```python
from build123d import *

# Parameters (mm, degrees)
SKETCH1_R           = 2.1
BOSS_EXTRUDE1_DEPTH = 3
CUT_EXTRUDE1_DEPTH  = 3
SKETCH3_R           = 5
SKETCH3_R_2         = 2.1
BOSS_EXTRUDE2_DEPTH = 6


with BuildPart() as part:
    # Sketch1 → Boss-Extrude1 (new, symmetric)
    with BuildSketch(Plane(origin=(0, 0, 0), x_dir=(1, 0, 0), z_dir=(0, 1, 0))):
        with BuildLine():
            Line((-5, 5), (5, 5))
            ThreePointArc((5, 5), (10, 0), (5, -5))
            Line((5, -5), (-5, -5))
            ThreePointArc((-5, -5), (-10, 0), (-5, 5))
        make_face()
        with Locations(Location((5, 0, 0), (0, 0, 270))):
            Circle(SKETCH1_R, mode=Mode.SUBTRACT)
        with Locations(Location((-5, 0, 0), (0, 0, 270))):
            Circle(SKETCH1_R, mode=Mode.SUBTRACT)
    extrude(amount=BOSS_EXTRUDE1_DEPTH, both=True)

    # Sketch2 → Cut-Extrude1 (cut)
    with BuildSketch(Plane(origin=(0, 3, 0), x_dir=(1, 0, 0), z_dir=(0, 1, 0))):
        Polygon((-9.041451884, 0), (-7.020725942, -3.5), (-2.979274058, -3.5), (-0.958548116, 0), (-2.979274058, 3.5), (-7.020725942, 3.5), align=None)
        Polygon((9.041451884, 0), (7.020725942, 3.5), (2.979274058, 3.5), (0.958548116, 0), (2.979274058, -3.5), (7.020725942, -3.5), align=None)
    extrude(amount=-CUT_EXTRUDE1_DEPTH, mode=Mode.SUBTRACT)

    # Sketch3 → Boss-Extrude2 (add)
    with BuildSketch(Plane.XZ.offset(3)):
        with Locations(Location((5, 0, 0), (0, 0, 270))):
            Circle(SKETCH3_R)
        with Locations(Location((5, 0, 0), (0, 0, 270))):
            Circle(SKETCH3_R_2, mode=Mode.SUBTRACT)
    extrude(amount=BOSS_EXTRUDE2_DEPTH)


solid = part.part
```
Here's how the part is built. I have some questions about the finished solid (model axes, mm). A direction names the side the tool comes from. Give positions to 0.01 mm unless a question says otherwise; leave off trailing zeros. Write each loop counter-clockwise with the first axis right and the second up, starting at its lowest first coordinate (ties: lowest second). Pieces come first, ordered by that corner, then holes. Notation, with made-up numbers: (-11.5, 80.25) -> (14.5, 80.25) arc R29 ccw to (14.5, 102.25) -> close; hole circle Ø11 at (84, 32.5). An arc over 180 degrees is marked (long way). Write each question's results on one line, items separated by ' | '.
Item 1: If I drill on L1, parallel to X at y = -0.85, z = 0; L2, parallel to Z at x = -5, y = -1.9; L3, parallel to X at y = 0.5, z = 0.75, over which ranges is the centre line in solid material (lowest first)?
Output:
L1: x = -10 to -7.1, -2.9 to 2.9, 7.1 to 10 | L2: z = -5 to -2.1, 2.1 to 5 | L3: x = -9.94 to -8.61, -1.39 to 1.39, 8.61 to 9.94
Item 2: Suppose I cut it at B-B on x = -4. Write out the boundary of the cut face in (y, z), plus the area to 3 significant figures.
Output:
outline: (-3, -5) -> (3, -5) -> (3, -3.5) -> (0, -3.5) -> (0, -1.85) -> (-3, -1.85) -> close; (-3, 1.85) -> (0, 1.85) -> (0, 3.5) -> (3, 3.5) -> (3, 5) -> (-3, 5) -> close | area: 27.9 mm^2
Item 3: For pin 1 Ø5 at (x, y) = (-1, -7) entering from -Z; pin 2 Ø1.5 at (y, z) = (-2.5, 3.5) entering from +X; pin 3 Ø5.5 at (x, z) = (-3, 0) entering from +Y; pin 4 Ø4 at (y, z) = (-2.5, 4) entering from +X, each with a flat end and sliding along its axis, tell me the tip position at first contact or that it passes through.
Output:
pin 1: stops at z = -3.57 | pin 2: stops at x = 9.18 | pin 3: stops at y = 3 | pin 4: stops at x = 9.58
Item 4: On a 3-axis mill with a long thin cutter (end or side, diameter ignored), from which of +Z, -Z, +X, -X, +Y, -Y can I reach the whole of each face in a straight line? I mean faces 5 (the face through (-5, 2, -3.5)), 6 (the face through (0, 0, 5)), 7 (the face through (9.957, -4.249, 0.651)). Say none if no direction works.
Output:
face 5: +Y | face 6: +Z, +X, -X, +Y, -Y | face 7: -Y
Item 5: Suppose I cut it at A-A on y = 1.5. Write out the boundary of the cut face in (x, z), plus the area to 3 significant figures.
Output:
outline: (-5, -5) -> (5, -5) arc R5 ccw to (5, 5) -> (-5, 5) arc R5 ccw to start; hole (-9.04, 0) -> (-7.02, -3.5) -> (-2.98, -3.5) -> (-0.96, 0) -> (-2.98, 3.5) -> (-7.02, 3.5) -> close; hole (0.96, 0) -> (2.98, -3.5) -> (7.02, -3.5) -> (9.04, 0) -> (7.02, 3.5) -> (2.98, 3.5) -> close | area: 93.7 mm^2
Item 6: Suppose I cut it at C-C on z = 1.25. Write out the boundary of the cut face in (x, y), plus the area to 3 significant figures.
Output:
outline: (-9.84, -3) -> (-6.69, -3) -> (-6.69, 0) -> (-8.32, 0) -> (-8.32, 3) -> (-9.84, 3) -> close; (-3.31, -3) -> (0.16, -3) -> (0.16, -9) -> (3.31, -9) -> (3.31, 0) -> (1.68, 0) -> (1.68, 3) -> (-1.68, 3) -> (-1.68, 0) -> (-3.31, 0) -> close; (6.69, -9) -> (9.84, -9) -> (9.84, 3) -> (8.32, 3) -> (8.32, 0) -> (6.69, 0) -> close | area: 95.9 mm^2
Item 7: Suppose I cut it at D-D on y = -6.25. Write out the boundary of the cut face in (x, z).
Output:
outline: circle Ø10 at (5, 0); hole circle Ø4.2 at (5, 0)
Item 8: We'd pull the mould along Z, two halves only. Please class faces 1 (the face through (-5, 2, 3.5)), 2 (the face through (-2, -3, 0)), 3 (the face through (-7.05, -1.52, -0.46)), 4 (the face through (0, 0, -5)): pulls with the +Z half, pulls with the -Z half, needs draft (parallel to the pull), parting line crosses it, or undercut.
Output:
face 1: undercut | face 2: needs draft | face 3: undercut | face 4: pulls with the -Z half
